Design review of the part built by this model. Coordinates are the model's own, in mm. A direction names the side the tool comes from. Round coordinates to 2 decimals unless told otherwise and drop trailing zeros. Write each loop counter-clockwise with the first axis right and the second up, starting at its lowest first coordinate (ties: lowest second). Pieces come first, ordered by that corner, then holes. Notation, with made-up numbers: (-30, -32.75) -> (3, -32.75) arc R20 cw to (3, -6.75) -> close; hole circle Ø11 at (17.5, 45). An arc over 180 degrees is marked (long way). One line per question, with ' | ' between items. Start each with the question number.
1) Consider section C-C (y = 1.9). Give the boundary of the cut face in (x, z), then the cut area to 3 significant figures.
2) Consider section A-A (z = 0). Give the boundary of the cut face in (x, y), then the cut area to 3 significant figures.
3) Consider section D-D (x = -26). Give the boundary of the cut face in (y, z).
4) Mouldability with a two-part tool opening along X and no side actions: class faces 3 (the flat face through (0, 1, -22.487)), 4 (the cylindrical face through (1.32, 1.48, -29.97)), 5 (the flat face through (-6, 0, 20)) as +X half, -X half, draft (parallel to the pull), parting line (faces both ways), or undercut.
5) For probe 1 along X at (y, z) = (1.55, 0); probe 2 along X at (y, z) = (2.6, -12.5); probe 3 along Z at (x, y) = (-11.5, 2.85), list the stretches that pass through material, from the lowest coordinate up.
6) Insertion check: pin 1 Ø1 at (y, z) = (1, -6.5) entering from -X; pin 2 Ø1 at (y, z) = (1.5, 21) entering from -X. Each pin has a flat end and moves straight along its axis. Give the tip position at first contact, or say it passes through.
7) Consider section B-B (x = 0). Give the boundary of the cut face in (y, z).
8) For faces 1 (the flat face through (0.75, 1, -21)), 2 (the flat face through (-6, 3, 20)), list the 3-axis set-ups (+Z, -Z, +X, -X, +Y, -Y) from which the entire face can be reached by the end or side of a thin tool; tool diameter is ignored.
```python
from build123d import *

# Parameters (mm, degrees)
ESQUISSE1_R        = 30
BOSS_EXTRU_1_DEPTH = 3


with BuildPart() as part:
    # Esquisse1 → Boss.-Extru.1 (new body)
    with BuildSketch(Plane(origin=(0, 0, 0), x_dir=(1, 0, 0), z_dir=(0, 1, 0))):
        with Locations(Location((0, 0, 0), (0, 0, 270))):
            Circle(ESQUISSE1_R)
        with BuildLine():
            Line((0.75, 22.487496526), (-0.75, 22.487496526))
            Line((-0.75, 22.487496526), (-0.75, 19.985932553))
            ThreePointArc((-0.75, 19.985932553), (0, -20), (0.75, 19.985932553))
            Line((0.75, 19.985932553), (0.75, 22.487496526))
        make_face(mode=Mode.SUBTRACT)
    extrude(amount=BOSS_EXTRU_1_DEPTH)


solid = part.part
```
From the geometry:
1) outline: circle Ø60 at (0, 0); hole (-0.75, -22.49) -> (0.75, -22.49) -> (0.75, -19.99) arc R20 ccw (long way) to (-0.75, -19.99) -> close | area: 1,570 mm2
2) outline: (-30, 0) -> (-20, 0) -> (-20, 3) -> (-30, 3) -> close; (20, 0) -> (30, 0) -> (30, 3) -> (20, 3) -> close | area: 60.0 mm2
3) outline: (0, -14.97) -> (3, -14.97) -> (3, 14.97) -> (0, 14.97) -> close
4) face 3: undercut | face 4: parting line | face 5: draft
5) probe 1: x = -30 to -20, 20 to 30 | probe 2: x = -27.27 to -15.61, 15.61 to 27.27 | probe 3: z = -27.71 to -16.36, 16.36 to 27.71
6) pin 1: stops at x = -29.39 | pin 2: stops at x = -21.9
7) outline: (0, -30) -> (3, -30) -> (3, -22.49) -> (0, -22.49) -> close; (0, 20) -> (3, 20) -> (3, 30) -> (0, 30) -> close
8) face 1: +Y, -Y | face 2: +Z, -Z, +X, -X, +Y
